Could you check a few things on this model? Use its own coordinates, in mm. A direction names the side the tool comes from. Give positions to 0.01 mm unless a question says otherwise; leave off trailing zeros. Order: outer loops, then holes, each group sorted by start corner. A loop starts at its lowest first (then second) coordinate and runs counter-clockwise, first axis right, second up. Notation, with made-up numbers: (81.25, 81) - (138.25, 81) arc R30 ccw to (138.25, 117) - close; hole circle Ø2 at (27.25, -34.5). An arc over 180 degrees is marked (long way). Put each result on its own line as item: value.
Autodesk Fusion 360 part; units mm, degrees
sketch "Sketch1" plane through (0, 0, 0) normal (0, 0, 1) x (1, 0, 0)
  line L0 (25.75, 36.6) -> (42.75, 36.6)
  line L1 (40.15, 44.6) -> (42.35, 44.6)
  line L2 (42.35, 44.6) -> (42.35, 40.4)
  line L3 (42.35, 40.4) -> (40.15, 40.4)
  line L4 (40.15, 40.4) -> (40.15, 44.6)
  line L5 (26.15, 40.4) -> (26.15, 44.6)
  line L6 (28.35, 44.6) -> (28.35, 40.4)
  line L7 (26.15, 44.6) -> (28.35, 44.6)
  line L8 (26.15, 40.4) -> (28.35, 40.4)
  line L9 (33.15, 48.6) -> (35.35, 48.6)
  line L10 (35.35, 48.6) -> (35.35, 44.4)
  line L11 (35.35, 44.4) -> (33.15, 44.4)
  line L12 (33.15, 44.4) -> (33.15, 48.6)
  line L13 (29.1351, 52.4) -> (39.36, 52.4)
  line L14 (22.75, 39.6) -> (22.75, 45.4272)
  line L15 (45.75, 39.6) -> (45.75, 45.3997)
  arc A0 (22.75, 39.6) -> (25.75, 36.6) centre (25.75, 39.6) ccw
  arc A1 (42.75, 36.6) -> (45.75, 39.6) centre (42.75, 39.6) ccw
  circle A2 centre (36.5318, 40.5854) radius 1.5
  circle A3 centre (31.9682, 40.5854) radius 1.5
  line L16 (23.4665, 47.3729) -> (26.8517, 51.3457)
  line L17 (45.0387, 47.3393) -> (41.6487, 51.3396)
  arc A4 (23.4665, 47.3729) -> (22.75, 45.4272) centre (25.75, 45.4272) ccw
  arc A5 (29.1351, 52.4) -> (26.8517, 51.3457) centre (29.1351, 49.4) ccw
  arc A6 (41.6487, 51.3396) -> (39.36, 52.4) centre (39.36, 49.4) ccw
  arc A7 (45.75, 45.3997) -> (45.0387, 47.3393) centre (42.75, 45.3997) ccw
  line L18 (28.85, 45.1) -> (28.85, 39.9)
  line L19 (25.65, 39.9) -> (28.85, 39.9)
  line L20 (25.65, 39.9) -> (25.65, 45.1)
  line L21 (25.65, 45.1) -> (28.85, 45.1)
  line L22 (35.85, 49.1) -> (35.85, 43.9)
  line L23 (35.85, 43.9) -> (32.65, 43.9)
  line L24 (32.65, 43.9) -> (32.65, 49.1)
  line L25 (32.65, 49.1) -> (35.85, 49.1)
  line L26 (42.85, 45.1) -> (42.85, 39.9)
  line L27 (42.85, 39.9) -> (39.65, 39.9)
  line L28 (39.65, 39.9) -> (39.65, 45.1)
  line L29 (39.65, 45.1) -> (42.85, 45.1)
  point P0 (22.75, 36.6)
  point P1 (45.75, 36.6)
  point P2 (27.75, 52.4)
  point P3 (40.75, 52.4)
  dimension "d1" = 23
  dimension "d22" = 13
  dimension "d29" = 3
  dimension "d31" = 3
  dimension "d32" = 3
  dimension "d34" = 3
  dimension "d35" = -0.5
  dimension "d36" = -0.5
  dimension "d37" = -0.5
extrude "Extrude1" add sketch "Sketch1" along normal blind 2 makes body 1 at (26.8833, 41.8, 0) makes body 2 at (33.8833, 47.2, 0) makes body 3 at (29.4506, 48.5152, 0) makes body 4 at (40.8833, 41.8, 0)
extrude "Extrude2" add sketch "Sketch1" along normal blind 11 contours L18 L19 L20 L21 | L22 L23 L24 L25 | L26 L27 L28 L29 bodies 1 2 3 4
extrude "Extrude5" add 1 faces at (25.8167, 43.2, 11) along direction (0, 0, 1) blind 1 on bodies 1 bodies 1
extrude "Extrude6" add 1 faces at (32.8167, 47.2, 11) along direction (0, 0, 1) blind 1 on bodies 1 bodies 1
extrude "Extrude7" add 1 faces at (42.6833, 41.8, 11) along direction (0, 0, 1) blind 1 on bodies 1 bodies 1
extrude "Extrude10" cut 1 faces at (33.8833, 47.2, 2) along direction (0, 0, -1) blind 1 on bodies 1 bodies 1
extrude "Extrude8" [suppressed]
extrude "Extrude3" [suppressed]
1) Suppose I cut it at A-A, the plane z = 8.5. List the corners of the cut face in (x, y) for me, and give its area (3 significant figures).
Filled in:
outline: (25.65, 39.9) - (28.85, 39.9) - (28.85, 45.1) - (25.65, 45.1) - close; (32.65, 43.9) - (35.85, 43.9) - (35.85, 49.1) - (32.65, 49.1) - close; (39.65, 39.9) - (42.85, 39.9) - (42.85, 45.1) - (39.65, 45.1) - close; hole (26.15, 40.4) - (28.35, 40.4) - (28.35, 44.6) - (26.15, 44.6) - close; hole (33.15, 44.4) - (35.35, 44.4) - (35.35, 48.6) - (33.15, 48.6) - close; hole (40.15, 40.4) - (42.35, 40.4) - (42.35, 44.6) - (40.15, 44.6) - close
area: 22.2 mm^2
2) We'd pull the mould along X, two halves only. Please class faces 6 (the flat face through (32.65, 46, 7)), 7 (the flat face through (28.85, 43, 7)), 8 (the flat face through (27, 39.9, 7)), 9 (the cylindrical face through (44.89, 37.5, 0.99)): pulls with the +X half, pulls with the -X half, needs draft (parallel to the pull), parting line crosses it, or undercut.
Filled in:
face 6: undercut
face 7: undercut
face 8: needs draft
face 9: pulls with the +X half
3) Suppose I cut it at B-B, the plane x = 32. List the corners of the cut face in (y, z) for me.
Filled in:
outline: (36.6, 0) - (39.09, 0) - (39.09, 2) - (36.6, 2) - close; (42.09, 0) - (52.4, 0) - (52.4, 2) - (42.09, 2) - close
4) Suppose I cut it at C-C, the plane y = 42.5. List the corners of the cut face in (x, z) for me, and give its area (3 significant figures).
Filled in:
outline: (22.75, 0) - (45.75, 0) - (45.75, 2) - (42.85, 2) - (42.85, 12) - (42.35, 12) - (42.35, 2) - (40.15, 2) - (40.15, 12) - (39.65, 12) - (39.65, 2) - (28.85, 2) - (28.85, 12) - (28.35, 12) - (28.35, 2) - (26.15, 2) - (26.15, 12) - (25.65, 12) - (25.65, 2) - (22.75, 2) - close
area: 66.0 mm^2
5) Suppose I cut it at D-D, the plane x = 34.75. List the corners of the cut face in (y, z) for me, and give its area (3 significant figures).
Filled in:
outline: (36.6, 0) - (52.4, 0) - (52.4, 2) - (49.1, 2) - (49.1, 12) - (48.6, 12) - (48.6, 1) - (44.4, 1) - (44.4, 12) - (43.9, 12) - (43.9, 2) - (36.6, 2) - close
area: 37.4 mm^2
6) If I drill on line 1 (X direction, y = 45, z = 8.25); line 2 (X direction, y = 42.25, z = 7.5); line 3 (Y direction, x = 34, z = 9.25), over which ranges is the centre line in solid material (lowest first)? Write a range as [from, to].
Filled in:
line 1: x = [25.65, 28.85], [32.65, 33.15], [35.35, 35.85], [39.65, 42.85]
line 2: x = [25.65, 26.15], [28.35, 28.85], [39.65, 40.15], [42.35, 42.85]
line 3: y = [43.9, 44.4], [48.6, 49.1]
7) Which directions (+Z, -Z, +X, -X, +Y, -Y) give clear straight access to the entire face, cutting with the end or side of a thin tool? Please do faces 1 (the flat face through (39.65, 42, 7)), 2 (the flat face through (25.65, 42, 7)), 3 (the flat face through (42.85, 43, 7)), 4 (the flat face through (34, 43.9, 7)), 5 (the flat face through (41, 40.4, 7)).
Filled in:
face 1: +Z, +Y, -Y
face 2: +Z, -X, +Y, -Y
face 3: +Z, +X, +Y, -Y
face 4: +Z, -Y
face 5: +Z
8) I'm going to push flat-ended pins straight in: pin 1 (1.6 mm diameter, centred on y = 45.5, z = 6, fed in from +X); pin 2 (1.1 mm diameter, centred on x = 41.5, z = 7, fed in from +Y); pin 3 (1.3 mm diameter, centred on y = 47, z = 4, fed in from +X). Where does each tip first touch, or does it pass through?
Filled in:
pin 1: stops at x = 42.85
pin 2: stops at y = 45.1
pin 3: stops at x = 35.85
